```python
from build123d import *

# Parameters (mm, degrees)
CYLINDER004_R          = 1.2
CYLINDER004_DEPTH      = 1.8
BOX014_W               = 64
BOX014_H               = 10
BOX014_DEPTH           = 15
FILLET005_R            = 2
CUT009_PLACEMENT_ANGLE = 90


with BuildPart() as array006:
    # Cylinder004 → Cylinder004 (new body)
    with BuildSketch(Plane(origin=(0, -50, 11.9), x_dir=(1, 0, 0), z_dir=(0, 0, 1))):
        Circle(CYLINDER004_R)
    extrude(amount=CYLINDER004_DEPTH)


with BuildPart() as obj1:
    # Box014 → Box014 (new body)
    with BuildSketch(Plane(origin=(-32, -55, -1.4), x_dir=(1, 0, 0), z_dir=(0, 0, 1))):
        with Locations((32, 5)):
            Rectangle(BOX014_W, BOX014_H)
    extrude(amount=BOX014_DEPTH)

    # Fillet005
    fillet005_edges = [obj1.edges().sort_by_distance(p)[0] for p in [
        (-32, -55, 6.1),
        (-32, -50, 13.6),
        (-32, -45, 6.1),
        (32, -55, 6.1),
        (32, -50, 13.6),
        (32, -45, 6.1),
        (0, -55, 13.6),
        (0, -45, 13.6),
    ]]
    fillet(fillet005_edges, radius=FILLET005_R)

    # Cut009: cut Array006
    add(array006.part, mode=Mode.SUBTRACT)


with BuildPart() as obj1_1:
    # Cut009 placement: moved
    add(obj1.part.moved(Location((-88, 0, -16))).rotate(Axis((-88, 0, -16), (0, 0, 1)), CUT009_PLACEMENT_ANGLE))


solid = obj1_1.part
```
Work out the finished part from the listing and answer in its coordinate system (mm). Round coordinates to 2 decimals unless told otherwise and drop trailing zeros. Write each loop counter-clockwise with the first axis right and the second up, starting at its lowest first coordinate (ties: lowest second). Pieces come first, ordered by that corner, then holes. Notation, with made-up numbers: (75.25, -23) - (101.25, -23) arc R26 cw to (101.25, 7) - close; hole circle Ø5 at (6.25, 75.5). An arc over 180 degrees is marked (long way). Return JSON: item names as keys, results as strings. Group by question number.
Q1. The mould has two halves that part along X. Classify faces 1 (the flat face through (-38, -32, -11)), 2 (the cylindrical face through (-33.57, 0.42, -3)), 3 (the cylindrical face through (-39.19, -0.16, -3.26)), 4 (the flat face through (-38, 0, -4.1)): released by +X, released by -X, zero draft, split by the parting line, or undercut.
Q2. Find the intervals of material crossed by L1, parallel to X at y = 0, z = -3.4; L2, parallel to Y at x = -38, z = -3.4; L3, parallel to X at y = 0, z = -3.5, in increasing order.
Q3. The part is cut by section A-A on y = 0. Write down the section's boundary in (x, z).
Q4. Each of these flat-tipped pins is pushed along its axis until it touches: pin 1 Ø1.5 at (x, y) = (-42, 8.5) entering from +Z; pin 2 Ø1.4 at (x, y) = (-38, 0) entering from +Z. Where does it stop, or does it pass through?
Solved:
{
 "1": {"face 1": "zero draft", "face 2": "released by +X", "face 3": "undercut", "face 4": "undercut"},
 "2": {"L1": "-42.73 to -39.2, -36.8 to -33.27", "L2": "-31.73 to -1.2, 1.2 to 31.73", "L3": "-42.79 to -39.2, -36.8 to -33.21"},
 "3": {"outline": "(-43, -17.4) - (-33, -17.4) - (-33, -4.4) arc R2 ccw to (-35, -2.4) - (-36.8, -2.4) - (-36.8, -4.1) - (-39.2, -4.1) - (-39.2, -2.4) - (-41, -2.4) arc R2 ccw to (-43, -4.4) - close"},
 "4": {"pin 1": "z = -2.42", "pin 2": "z = -4.1"}
}
